from build123d import *

# Parameters (mm, degrees)
F0_W     = 400
F0_H     = 400
F1_DEPTH = 50.8
F2_SIZE  = 50
F3_W     = 152.4
F3_H     = 152.4
F4_DEPTH = 520.7


with BuildPart() as f1:
    # F0 (on Top) → F1 (new body)
    with BuildSketch(Plane.XY):
        Rectangle(F0_W, F0_H)
    extrude(amount=F1_DEPTH)

    # F2
    f2_edges = [f1.edges().sort_by_distance(p)[0] for p in [
        (-200, 200, 25.4),
        (-200, -200, 25.4),
        (200, -200, 25.4),
        (200, 200, 25.4),
    ]]
    chamfer(f2_edges, length=F2_SIZE)

    # F3 (on face) → F4 (join)
    with BuildSketch(Plane.XY.offset(50.8)):
        Rectangle(F3_W, F3_H)
    extrude(amount=F4_DEPTH)


solid = f1.part
The model under review builds one solid part; all positions refer to its coordinate system, in mm. A direction names the side the tool comes from. Coordinates: 2 decimals unless noted, no trailing zeros. Loops run counter-clockwise (first coordinate to the right, second up) from the corner with the lowest first, then second, coordinate; pieces in that order, holes last. Notation, with made-up numbers: (78, -30.75) -> (96, -30.75) arc R33 ccw to (96, 7.25) -> close; hole circle Ø1 at (81.25, 33.25). An arc over 180 degrees is marked (long way). Use a Markdown table: item, result. Add a question column.
1. Add section D-D on x = 161. Write out the cut boundary in (y, z), plus the area to 3 significant figures.
2. Add section C-C on z = 483. Write out the cut boundary in (x, y).
3. Machinability: for faces 1 (the face through (-1, 76.2, 308)), 2 (the face through (-1, -76.2, 308)), 3 (the face through (-76.2, -1, 308)), 4 (the face through (76.2, -1, 308)), which of the approach directions +Z, -Z, +X, -X, +Y, -Y give a long, thin tool a straight path to every point of the face, cutting with its end or side? Answer none if there is none.
4. To check wall thickness, follow line 1 (Z direction, x = -96.5, y = 178.5); line 2 (X direction, y = 16.5, z = 103). State the ranges of each line that lie inside material, in increasing order.
5. Add section A-A on x = 26. Write out the cut boundary in (y, z), plus the area to 3 significant figures.
6. Clearance check with flat-ended pins moving along their axes: pin 1 Ø6 at (y, z) = (44, 122) entering from -X; pin 2 Ø1 at (x, z) = (59.5, 217.5) entering from +Y; pin 3 Ø3 at (x, z) = (41, 250) entering from -Y. State where each tip first meets the part, or that it passes through.
Returned:
| question | item | result |
|---|---|---|
| 1 | outline | (-189, 0) -> (189, 0) -> (189, 50.8) -> (-189, 50.8) -> close |
| 1 | area | 19,200 mm² |
| 2 | outline | (-76.2, -76.2) -> (76.2, -76.2) -> (76.2, 76.2) -> (-76.2, 76.2) -> close |
| 3 | face 1 | +Z, +X, -X, +Y |
| 3 | face 2 | +Z, +X, -X, -Y |
| 3 | face 3 | +Z, -X, +Y, -Y |
| 3 | face 4 | +Z, +X, +Y, -Y |
| 4 | line 1 | z = 0 to 50.8 |
| 4 | line 2 | x = -76.2 to 76.2 |
| 5 | outline | (-200, 0) -> (200, 0) -> (200, 50.8) -> (76.2, 50.8) -> (76.2, 571.5) -> (-76.2, 571.5) -> (-76.2, 50.8) -> (-200, 50.8) -> close |
| 5 | area | 99,700 mm² |
| 6 | pin 1 | stops at x = -76.2 |
| 6 | pin 2 | stops at y = 76.2 |
| 6 | pin 3 | stops at y = -76.2 |
